from build123d import *

# Parameters (mm, degrees)
F0_R     = 14.3891
F0_R_2   = 12.7
F1_DEPTH = 50.8
F2_R     = 14.3891
F2_R_2   = 12.7
F3_DEPTH = 50.8
F4_R     = 14.3891
F4_R_2   = 12.7
F5_DEPTH = 50.8


with BuildPart() as f1:
    # F0 (on Front) → F1 (new body)
    with BuildSketch(Plane.XZ):
        Circle(F0_R)
        Circle(F0_R_2, mode=Mode.SUBTRACT)
    extrude(amount=F1_DEPTH)

    # F2 (on Right) → F3 (join)
    with BuildSketch(Plane.YZ):
        Circle(F2_R)
        Circle(F2_R_2, mode=Mode.SUBTRACT)
    extrude(amount=F3_DEPTH)

    # F4 (on Top) → F5 (join)
    with BuildSketch(Plane.XY):
        Circle(F4_R)
        Circle(F4_R_2, mode=Mode.SUBTRACT)
    extrude(amount=F5_DEPTH)

    # F6 (on Front) → F7 (revolve)
    with BuildSketch(Plane.XZ):
        with BuildLine():
            ThreePointArc((14.3891, 0), (0, 14.3891), (-14.3891, 0))
            Line((-14.3891, 0), (14.3891, 0))
        make_face()
    revolve(axis=Axis((0, 0, 0), (1, 0, 0)))


solid = f1.part
For this review, take the finished solid that the model builds, in its own axes (mm). A direction names the side the tool comes from. Round coordinates to 2 decimals unless told otherwise and drop trailing zeros. Write each loop counter-clockwise with the first axis right and the second up, starting at its lowest first coordinate (ties: lowest second). Pieces come first, ordered by that corner, then holes. Notation, with made-up numbers: (-22.75, -17.5) -> (-2.75, -17.5) arc R6 ccw to (-2.75, -10.5) -> close; hole circle Ø8 at (68.25, -6.5). An arc over 180 degrees is marked (long way). Put each result on its own line as item: value.
Q1. Machinability: for faces 4 (the cylindrical face through (-9.36, 8.583, 28.474)), 5 (the cylindrical face through (-10.1, -28.5, -7.7)), 6 (the cylindrical face through (10.22, -2.9, 10.13)), which of the approach directions +Z, -Z, +X, -X, +Y, -Y give a long, thin tool a straight path to every point of the face, cutting with its end or side? Answer none if there is none.
Determined:
face 4: +Z
face 5: -Y
face 6: none
Q2. Clearance check with flat-ended pins moving along their axes: pin 1 Ø1.5 at (x, z) = (19, 14) entering from -Y; pin 2 Ø10 at (y, z) = (-16, 15) entering from -X; pin 3 Ø10 at (y, z) = (-0.5, 37) entering from +X; pin 4 Ø8 at (x, y) = (15, 5) entering from +Z. State where each tip first meets the part, or that it passes through.
Determined:
pin 1: stops at y = -5.61
pin 2: stops at x = -10.35
pin 3: stops at x = 14.39
pin 4: stops at z = 50.8
Q3. Consider section A-A on x = 46. State the section outline as (y, z) points.
Determined:
outline: circle Ø28.78 at (0, 0); hole circle Ø25.4 at (0, 0)
Q4. The part is to be moulded in two halves that separate along X. For faces 1 (the cylindrical face through (-11.419, -30.689, -8.756)), 2 (the cylindrical face through (30.689, 13.292, -5.511)), 3 (the cylindrical face through (9.69, -12.51, -2.18)), say which applies: released by +X, released by -X, zero draft, split by the parting line, or undercut.
Determined:
face 1: split by the parting line
face 2: zero draft
face 3: undercut
Q5. Consider section C-C on z = -2. State the section outline as (x, y) points.
Determined:
outline: (-14.25, -50.8) -> (-12.54, -50.8) -> (-12.54, -6.76) arc R14.25 ccw to (0, -14.25) -> (12.54, -14.25) -> (12.54, -50.8) -> (14.25, -50.8) -> (14.25, -14.25) -> (50.8, -14.25) -> (50.8, -12.54) -> (14.25, -12.54) -> (14.25, 0) arc R14.25 ccw to (6.76, 12.54) -> (50.8, 12.54) -> (50.8, 14.25) -> (0, 14.25) arc R14.25 ccw to (-14.25, 0) -> close; hole (6.76, -12.54) -> (12.54, -12.54) -> (12.54, -6.76) arc R14.25 cw to start
Q6. To check wall thickness, follow L1, parallel to Y at x = 32, z = 0; L2, parallel to Y at x = 8, z = -7.5. State the ranges of each line that lie inside material, in increasing order. Write a range as [from, to].
Determined:
L1: y = [-14.39, -12.7], [12.7, 14.39]
L2: y = [-12.28, -10.25], [-9.32, 9.32], [10.25, 12.28]
